```python
from build123d import *

# Parameters (mm, degrees)
F0_W     = 14
F0_H     = 27
F1_DEPTH = 4
F2_R     = 1
F4_DEPTH = 4
F5_DEPTH = 4
F6_DEPTH = 1.5


with BuildPart() as f1:
    # F0 (on Top) → F1 (new body)
    with BuildSketch(Plane.XY):
        with Locations((7, 13.5)):
            Rectangle(F0_W, F0_H)
    extrude(amount=F1_DEPTH)

    # F2 (on face) → F3 (revolve, cut)
    with BuildSketch(Plane.XY.offset(4)):
        with BuildLine():
            ThreePointArc((7, 14.75), (12.25, 20), (7, 25.25))
            Line((7, 25.25), (7, 14.75))
        make_face()
    revolve(axis=Axis((7, 20, 4), (0, -1, 0)), mode=Mode.SUBTRACT)

    # F2 (on face) → F4 (cut)
    with BuildSketch(Plane.XY.offset(4)):
        with Locations((2, 25)):
            Circle(F2_R)
        with Locations((12, 14.5)):
            Circle(F2_R)
        with Locations((12, 25)):
            Circle(F2_R)
        with Locations((2, 14.5)):
            Circle(F2_R)
    extrude(amount=-F4_DEPTH, mode=Mode.SUBTRACT)

    # F2 (on face) → F5 (cut)
    with BuildSketch(Plane.XY.offset(4)):
        Polygon((2.15, 12), (2.15, 8), (4.15, 8), (4.15, 7.25), (6.15, 7.25), (6.15, 6.25), (4.15, 6.25), (4.15, 2.75), (6.15, 2.75), (6.15, 0.75), (4.15, 0.75), (4.15, 0), (9.85, 0), (9.85, 0.75), (7.85, 0.75), (7.85, 2.75), (9.85, 2.75), (9.85, 6.25), (7.85, 6.25), (7.85, 7.25), (9.85, 7.25), (9.85, 8), (11.85, 8), (11.85, 12), align=None)
    extrude(amount=-F5_DEPTH, mode=Mode.SUBTRACT)

    # F2 (on face) → F6 (cut)
    with BuildSketch(Plane.XY.offset(4)):
        Polygon((2.15, 8), (2.15, 0), (4.15, 0), (4.15, 0.75), (6.15, 0.75), (6.15, 2.75), (4.15, 2.75), (4.15, 6.25), (6.15, 6.25), (6.15, 7.25), (4.15, 7.25), (4.15, 8), align=None)
        Polygon((9.85, 0.75), (9.85, 0), (11.85, 0), (11.85, 8), (9.85, 8), (9.85, 7.25), (7.85, 7.25), (7.85, 6.25), (9.85, 6.25), (9.85, 2.75), (7.85, 2.75), (7.85, 0.75), align=None)
    extrude(amount=-F6_DEPTH, mode=Mode.SUBTRACT)


solid = f1.part
```
The listing builds one solid part. Answer for the finished solid, in the listing's coordinates (mm). A direction names the side the tool comes from. Give positions to 0.01 mm unless a question says otherwise; leave off trailing zeros. Write each loop counter-clockwise with the first axis right and the second up, starting at its lowest first coordinate (ties: lowest second). Pieces come first, ordered by that corner, then holes. Notation, with made-up numbers: (-4.75, -1) -> (48.25, -1) arc R8 ccw to (48.25, 6) -> close; hole circle Ø2 at (8, 63.5). An arc over 180 degrees is marked (long way). Use one line per item in the form item = value.
1) Section B-B on x = 6.5 is taken. Write down the section's boundary in (y, z), plus the area to 3 significant figures.
Result:
outline = (12, 0) -> (16.64, 0) arc R5.23 cw to (14.77, 4) -> (12, 4) -> close; (23.36, 0) -> (27, 0) -> (27, 4) -> (25.23, 4) arc R5.23 cw to start
area = 22.7 mm²
2) Straight lines are drawn through the part: probe 1 along Y at (x, z) = (12, 1.9); probe 2 along X at (y, z) = (6.25, 3.6); probe 3 along Y at (x, z) = (8.5, 0.5). For each, find the intervals that lie inside material, in ascending order.
Result:
probe_1 = 0 to 13.5, 15.5 to 24, 26 to 27
probe_2 = 0 to 2.15, 11.85 to 14
probe_3 = 0.75 to 2.75, 6.25 to 7.25, 12 to 16.39, 23.61 to 27
3) Section D-D on z = 3.1 is taken. Write down the section's boundary in (x, y).
Result:
outline = (0, 0) -> (2.15, 0) -> (2.15, 12) -> (11.85, 12) -> (11.85, 0) -> (14, 0) -> (14, 27) -> (0, 27) -> close; hole circle Ø2 at (2, 14.5); hole circle Ø2 at (2, 25); hole circle Ø10.34 at (7, 20); hole circle Ø2 at (12, 14.5); hole circle Ø2 at (12, 25)
4) A tool of negligible diameter and unlimited length cuts with its end or side. For faces 5 (the flat face through (0, 13, 2)), 6 (the flat face through (11, 8, 1)), 7 (the flat face through (6.15, 7, 1)), from which of +Z, -Z, +X, -X, +Y, -Y can it reach the whole face along a straight path? Write none if from no direction.
Result:
face_5 = +Z, -Z, -X, +Y, -Y
face_6 = +Z, -Z
face_7 = +Z, -Z, -Y
5) Section A-A on y = 10.25 is taken. Write down the section's boundary in (x, z), plus the area to 3 significant figures.
Result:
outline = (0, 0) -> (2.15, 0) -> (2.15, 4) -> (0, 4) -> close; (11.85, 0) -> (14, 0) -> (14, 4) -> (11.85, 4) -> close
area = 17.2 mm²
6) For a pull along Y with two mould halves and no side action, classify faces 1 (the flat face through (7, 27, 2)), 2 (the flat face through (11.85, 7, 3)), 3 (the flat face through (2, 0, 2)), 4 (the flat face through (10, 4, 2.5)) as +Y half, -Y half, draft (parallel to the pull), parting line (faces both ways), or undercut.
Result:
face_1 = +Y half
face_2 = undercut
face_3 = -Y half
face_4 = draft
7) Section C-C on y = 14.5 is taken. Write down the section's boundary in (x, z), plus the area to 3 significant figures.
Result:
outline = (0, 0) -> (1, 0) -> (1, 4) -> (0, 4) -> close; (3, 0) -> (11, 0) -> (11, 4) -> (3, 4) -> close; (13, 0) -> (14, 0) -> (14, 4) -> (13, 4) -> close
area = 40.0 mm²
8) Each of these flat-tipped pins is pushed along its axis until it touches: P1, Ø1.6, axis at x = 5.5, z = 1.5, coming from the -Y side; P2, Ø3, axis at x = 9.5, y = 5.5, coming from the +Z side; P3, Ø1.6, axis at x = 12, y = 25, coming from the -Z side. Where does it stop, or does it pass through?
Result:
P1 = 0.75
P2 = 2.5
P3 = through
